Build history of the part. All positions in model axes, mm. A direction names the side the tool comes from. Give positions to 0.01 mm unless a question says otherwise; leave off trailing zeros. Loops run counter-clockwise (first coordinate to the right, second up) from the corner with the lowest first, then second, coordinate; pieces in that order, holes last.
1) Two-plate mould, pull along X, no slides. Class faces 1 (the flat face through (-3, -5, 19.05)), 2 (the cylindrical face through (0.083, 3.968, 9.409)): +X half, -X half, draft (parallel to the pull), parting line (faces both ways), or undercut.
2) Wall check: line 1 (Y direction, x = 8, z = 2.5); line 2 (Y direction, x = -9.75, z = 10.25); line 3 (X direction, y = 2.5, z = 3.5). Give the ranges that are in metal, low to high.
3) Band-saw the part on C-C on y = -8.25. List the corners of the cut face in (x, z).
4) 3-axis set-ups, long thin cutter, end or side, ignore diameter. For faces 3 (the flat face through (-8, 0.318, 10)), 4 (the cylindrical face through (-0.083, -3.968, 9.409)), 5 (the flat face through (-3, -5, 0)): which of +Z, -Z, +X, -X, +Y, -Y reach the whole face in a straight line?
5) Flat gauge pins, fed straight in: P1, Ø5.5, axis at x = -6.5, z = 12, coming from the -Y side; P2, Ø2, axis at y = 5, z = 6.5, coming from the +X side; P3, Ø1.5, axis at x = -3, y = 3, coming from the +Z side. Where does each tip first touch, or does it go through?
6) Band-saw the part on A-A on x = 0. List the corners of the cut face in (y, z).
7) Band-saw the part on B-B on z = 8. List the corners of the cut face in (x, y), then the cut area to 3 significant figures.
```python
from build123d import *

# Parameters (mm, degrees)
SKETCH1_R           = 11.049
SKETCH1_R_2         = 3.96875
BOSS_EXTRUDE1_DEPTH = 19.05
FILLET1_R           = 1.27
SKETCH3_W           = 21.529859436
SKETCH3_H           = 0.635
CUT_EXTRUDE1_DEPTH  = 20.05


with BuildPart() as part:
    # Sketch1 → Boss-Extrude1 (new body)
    with BuildSketch(Plane.XY):
        Circle(SKETCH1_R)
        Circle(SKETCH1_R_2, mode=Mode.SUBTRACT)
    extrude(amount=BOSS_EXTRUDE1_DEPTH)

    # Fillet1
    fillet1_edges = [part.edges().sort_by_distance(p)[0] for p in [
        (-3.96875, 0, 0),
        (-3.96875, 0, 19.05),
    ]]
    fillet(fillet1_edges, radius=FILLET1_R)

    # Sketch3 → Cut-Extrude1 (cut, through all)
    with BuildSketch(Plane.XY.offset(19.05)):
        with Locations((-0.784069021, 0)):
            Rectangle(SKETCH3_W, SKETCH3_H)
    extrude(amount=-CUT_EXTRUDE1_DEPTH, mode=Mode.SUBTRACT)


solid = part.part
```
Findings below:
1. face 1: draft
1. face 2: undercut
2. line 1: y = -7.62 to -0.32, 0.32 to 7.62
2. line 2: y = -5.2 to -0.32, 0.32 to 5.2
2. line 3: x = -10.76 to -3.08, 3.08 to 10.76
3. outline: (-7.35, 0) - (7.35, 0) - (7.35, 19.05) - (-7.35, 19.05) - close
4. face 3: +Z, -Z, -X
4. face 4: +Z, -Z
4. face 5: -Z, +X, -X, +Y, -Y
5. P1: stops at y = -10.39
5. P2: stops at x = 10.3
5. P3: stops at z = 19.03
6. outline: (-11.05, 0) - (-5.24, 0) arc R1.27 ccw to (-3.97, 1.27) - (-3.97, 17.78) arc R1.27 ccw to (-5.24, 19.05) - (-11.05, 19.05) - close; (3.97, 1.27) arc R1.27 ccw to (5.24, 0) - (11.05, 0) - (11.05, 19.05) - (5.24, 19.05) arc R1.27 ccw to (3.97, 17.78) - close
7. outline: (-11.04, -0.32) arc R11.05 ccw (long way) to (-11.04, 0.32) - (-3.96, 0.32) arc R3.97 cw to (3.96, 0.32) - (9.98, 0.32) - (9.98, -0.32) - (3.96, -0.32) arc R3.97 cw to (-3.96, -0.32) - close
7. area: 326 mm2
